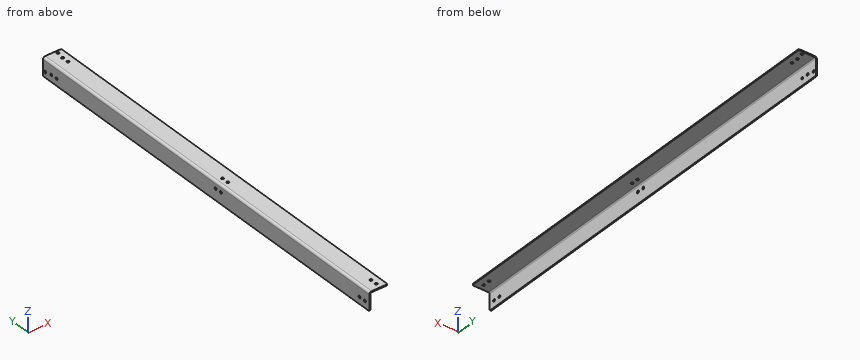
```python
from build123d import *

# Parameters (mm, degrees)
BASE_FLANGE1_DEPTH = 1159.383
SKETCH2_R          = 3.429
CUT_EXTRUDE1_DEPTH = 3.175
SKETCH3_R          = 3.429
CUT_EXTRUDE2_DEPTH = 3.175
FILLET1_R          = 3.175


# Sheet-metal steps are written as plain solids
with BuildPart() as part:
    # Sketch1 → Base-Flange1 (new body)
    with BuildSketch(Plane(origin=(0, 0, 0), x_dir=(1, 0, 0), z_dir=(0, 1, 0))):
        with BuildLine():
            Line((0, 50.8), (0, 6.35))
            ThreePointArc((0, 6.35), (1.859871939, 1.859871939), (6.35, 0))
            Line((6.35, 0), (50.8, 0))
            Line((50.8, 0), (50.8, 3.175))
            Line((50.8, 3.175), (6.35, 3.175))
            ThreePointArc((6.35, 3.175), (4.10493597, 4.10493597), (3.175, 6.35))
            Line((3.175, 6.35), (3.175, 50.8))
            Line((3.175, 50.8), (0, 50.8))
        make_face()
    extrude(amount=BASE_FLANGE1_DEPTH)

    # Sketch2 → Cut-Extrude1 (cut)
    with BuildSketch(Plane.XY):
        with Locations((31.75, 34.925)):
            Circle(SKETCH2_R)
        with Locations((31.75, 15.875)):
            Circle(SKETCH2_R)
        with Locations((19.05, 546.1)):
            Circle(SKETCH2_R)
        with Locations((19.05, 527.05)):
            Circle(SKETCH2_R)
        with Locations((31.75, 1130.173)):
            Circle(SKETCH2_R)
        with Locations((31.75, 1111.123)):
            Circle(SKETCH2_R)
        with Locations((35.56, 1151.4455)):
            Circle(SKETCH2_R)
    extrude(amount=-CUT_EXTRUDE1_DEPTH, mode=Mode.SUBTRACT)

    # Sketch3 → Cut-Extrude2 (cut)
    with BuildSketch(Plane.ZY):
        with Locations((-35.56, 1151.4455)):
            Circle(SKETCH3_R)
        with Locations((-31.75, 34.925)):
            Circle(SKETCH3_R)
        with Locations((-31.75, 15.875)):
            Circle(SKETCH3_R)
        with Locations((-19.05, 546.1)):
            Circle(SKETCH3_R)
        with Locations((-19.05, 527.05)):
            Circle(SKETCH3_R)
        with Locations((-31.75, 1130.173)):
            Circle(SKETCH3_R)
        with Locations((-31.75, 1111.123)):
            Circle(SKETCH3_R)
    extrude(amount=-CUT_EXTRUDE2_DEPTH, mode=Mode.SUBTRACT)

    # Fillet1
    fillet1_edges = [part.edges().sort_by_distance(p)[0] for p in [
        (1.5875, 1159.383, -50.8),
        (1.5875, 0, -50.8),
        (50.8, 1159.383, -1.5875),
        (50.8, 0, -1.5875),
    ]]
    fillet(fillet1_edges, radius=FILLET1_R)


solid = part.part
```
Geometry check sheet. Reference: the model listing, model coordinates, mm. Round coordinates to 2 decimals unless told otherwise and drop trailing zeros. Order: outer loops, then holes, each group sorted by start corner. A loop starts at its lowest first (then second) coordinate and runs counter-clockwise, first axis right, second up. Notation, with made-up numbers: M -3,28.5 L 35,28.5 A29 cw 35,67.5 Z; hole C 26.5,34 d2. An arc over 180 degrees is marked long. Answer as CSV lines item,"result".
1) Thickness scan on probe 1 along Y at (x, z) = (1.1, -31.75); probe 2 along Y at (x, z) = (19, -1); probe 3 along Y at (x, z) = (31, -1). Record the ranges inside material, lowest first. Write a range as [from, to].
Entries:
probe 1,"[0, 12.45], [19.3, 31.5], [38.35, 1107.69], [1114.55, 1126.74], [1133.6, 1159.38]"
probe 2,"[0, 523.62], [530.48, 542.67], [549.53, 1159.38]"
probe 3,"[0, 12.53], [19.22, 31.58], [38.27, 1107.78], [1114.47, 1126.83], [1133.52, 1159.38]"
2) Sectioned sample at A-A on y = 775.5. Record the cut outline in (x, z) (3 decimals), and give its area (3 significant figures).
Entries:
outline,"M 0,-50.8 L 3.175,-50.8 L 3.175,-6.35 A3.175 cw 6.35,-3.175 L 50.8,-3.175 L 50.8,0 L 6.35,0 A6.35 ccw 0,-6.35 Z"
area,"306 mm2"
3) Gauge pin test, flat ends, axial feed: pin 1 Ø9 at (x, y) = (31.75, 34.925) entering from -Z (3 decimals); pin 2 Ø11 at (y, z) = (15.875, -31.75) entering from +X (3 decimals). Record the tip position at first contact, or that the pin passes through.
Entries:
pin 1,"z = -3.175"
pin 2,"x = 3.175"
